```python
from build123d import *

# Parameters (mm, degrees)
F0_W             = 20
F0_H             = 20
F1_DEPTH         = 463
F2_R             = 2.1
F3_DEPTH         = 463.001
F4_R             = 1
F6_DEPTH         = 463.001
F6_COPIES3_COUNT = 2
F6_COPIES3_ANGLE = 90
F6_COPIES4_COUNT = 2
F6_COPIES4_ANGLE = 270
F6_COPIES6_COUNT = 2
F9_W             = 16.4
F9_H             = 6.8613203436
F10_DEPTH        = 463.001
F12_DEPTH        = 463


# Not quite as in the source:
# - a pattern or mirror of a feature is missing from the dataset's text; its kind, count and spacing are read off the source's solid


with BuildPart() as f1:
    # F0 (on Front) → F1 (new body)
    with BuildSketch(Plane.XZ):
        Rectangle(F0_W, F0_H)
    extrude(amount=F1_DEPTH)

    # F2 (on face) → F3 (cut, through all)
    with BuildSketch(Plane.XZ.offset(463)):
        Circle(F2_R)
    extrude(amount=-F3_DEPTH, mode=Mode.SUBTRACT)

    # F4
    f4_edges = [f1.edges().sort_by_distance(p)[0] for p in [
        (-10, -231.5, 10),
        (10, -231.5, 10),
    ]]
    fillet(f4_edges, radius=F4_R)

    # F5 (on face) → F6 (cut, through all)
    with BuildSketch(Plane.XZ.offset(463)):
        Polygon((0, 3.9006601718), (0, 10), (-2.84, 10), (-4.64, 10), (-2.84, 8.2), (-5.4993398282, 8.2), (-5.4993398282, 6.56), (-2.84, 3.9006601718), align=None)
        Polygon((-6.5693398282, 8.2), (-8.2, 8.2), (-7.0953059148, 7.0953059148), (-6.5693398282, 7.6212720014), align=None)
    f6 = extrude(amount=-F6_DEPTH, mode=Mode.SUBTRACT)

    # F6_copies: F6 across plane
    add(f6.mirror(Plane(origin=(0, 0, 0), x_dir=(-0.7071067812, 0, -0.7071067812), z_dir=(0.7071067812, 0, -0.7071067812))), mode=Mode.SUBTRACT)

    # F6_copies1: F6 across plane
    add(f6.mirror(Plane(origin=(0, 0, 0), x_dir=(0.7071067812, 0, -0.7071067812), z_dir=(-0.7071067812, 0, -0.7071067812))), mode=Mode.SUBTRACT)

    # F6_copies2: F6 across plane
    add(f6.mirror(Plane(origin=(0, 0, 0), x_dir=(0, 0, 1), z_dir=(1, 0, 0))), mode=Mode.SUBTRACT)

    # F6_copies3: F6 ×2 about axis
    f6_copies3_axis = Axis((0, 0, 0), (0, 1, 0))
    for i in range(1, F6_COPIES3_COUNT):
        add(f6.rotate(f6_copies3_axis, i * F6_COPIES3_ANGLE / (F6_COPIES3_COUNT - 1)), mode=Mode.SUBTRACT)

    # F6_copies4: F6 ×2 about axis
    f6_copies4_axis = Axis((0, 0, 0), (0, 1, 0))
    for i in range(1, F6_COPIES4_COUNT):
        add(f6.rotate(f6_copies4_axis, i * F6_COPIES4_ANGLE / (F6_COPIES4_COUNT - 1)), mode=Mode.SUBTRACT)

    # F6_copies5: F6 across plane
    add(f6.mirror(Plane(origin=(0, 0, 0), x_dir=(-1, 0, 0), z_dir=(0, 0, -1))), mode=Mode.SUBTRACT)

    # F6_copies6: F6 ×2 about axis
    f6_copies6_axis = Axis((0, 0, 0), (0, 1, 0))
    for i in range(1, F6_COPIES6_COUNT):
        add(f6.rotate(f6_copies6_axis, i * 360 / F6_COPIES6_COUNT), mode=Mode.SUBTRACT)

    # F8: F1 across face


with BuildPart() as f1_1:
    add(f1.part)
    add(f1.part.mirror(Plane(origin=(-7.32, -231.5, -10), x_dir=(1, 0, 0), z_dir=(0, 0, -1))))

    # F9 (on face) → F10 (cut, through all)
    with BuildSketch(Plane.XZ.offset(463)):
        with Locations((0, -10)):
            Rectangle(F9_W, F9_H)
    extrude(amount=-F10_DEPTH, mode=Mode.SUBTRACT)

    # F11 (on face) → F12 (join, through all)
    with BuildSketch(Plane.XZ.offset(463)):
        with BuildLine():
            ThreePointArc((-9, -10), (-9.7071067812, -9.7071067812), (-10, -9))
            Line((-10, -9), (-10, -11))
            ThreePointArc((-10, -11), (-9.7071067812, -10.2928932188), (-9, -10))
        make_face()
        with BuildLine():
            ThreePointArc((10, -9), (9.7071067812, -9.7071067812), (9, -10))
            ThreePointArc((9, -10), (9.7071067812, -10.2928932188), (10, -11))
            Line((10, -11), (10, -9))
        make_face()
        Polygon((5.9386796564, -6.9993398282), (8.2, -6.9993398282), (8.2, -6.5693398282), (5.5086796564, -6.5693398282), align=None)
        Polygon((-8.2, -6.5693398282), (-8.2, -6.9993398282), (-5.9386796564, -6.9993398282), (-5.5086796564, -6.5693398282), align=None)
    extrude(amount=-F12_DEPTH)


solid = f1_1.part
```
Build history of the part. All positions in model axes, mm. Give positions to 0.01 mm unless a question says otherwise; leave off trailing zeros.
1) Drop flat-ended pins along their axis: P1, Ø1.7, axis at x = 0.5, y = -278, coming from the -Z side; P2, Ø0.8, axis at y = -178.5, z = 4, coming from the +X side; P3, Ø2, axis at x = -3.5, y = -215, coming from the -Z side. Give the stop position or say it passes through.
Values follow:
P1: stops at z = -23.9
P2: stops at x = 9.76
P3: stops at z = -29.86
2) Band-saw the part on A-A on y = -415. State how many separate pieces and enclosed holes the cut face has, then the cut area to 3 significant figures.
Values follow:
separate pieces: 1
enclosed holes: 7
area: 286 mm2
3) Probe line 1 along Z through (x, y) = (-6.5, -139); line 2 along Z through (x, y) = (0, -186); line 3 along X through (y, z) = (-283, -17). List the from-to ranges inside material, lowest first.
Values follow:
line 1: z = -30 to -25.44, -14.56 to -13.43, -7 to -5.44, 5.44 to 10
line 2: z = -23.9 to -22.1, -17.9 to -16.1, -3.9 to -2.1, 2.1 to 3.9
line 3: x = -8.36 to -8.2, -4.06 to 4.06, 8.2 to 8.36
